```python
from build123d import *

# Parameters (mm, degrees)
BOSS_EXTRUDE1_DEPTH      = 3.175
BOSS_EXTRUDE1_DEPTH_BACK = 3.175
SKETCH1_R                = 4.178670833


with BuildPart() as part:
    # Sketch1 → Boss-Extrude1 (new, two sides: drawn at the far end of the back side and taken through both)
    with BuildSketch(Plane.XY.offset(-BOSS_EXTRUDE1_DEPTH_BACK)):
        with BuildLine():
            Line((596.301932932, 140.061825094), (593.775672351, 134.913286528))
            Line((593.775672351, 134.913286528), (596.301932932, 127.519508045))
            Line((596.301932932, 127.519508045), (596.301932932, 112.761180415))
            Line((596.301932932, 112.761180415), (620.507043959, 121.0314333))
            Line((620.507043959, 121.0314333), (621.935426787, 129.559046913))
            ThreePointArc((621.935426787, 129.559046913), (624.139317927, 134.860628873), (628.452705625, 138.649902417))
            ThreePointArc((628.452705625, 138.649902417), (629.422874429, 139.237084375), (630.327572389, 139.920847318))
            Line((630.327572389, 139.920847318), (641.475190915, 144.713939185))
            Line((641.475190915, 144.713939185), (645.828084101, 149.293372969))
            Line((645.828084101, 149.293372969), (645.073577651, 155.192660049))
            Line((645.073577651, 155.192660049), (642.120102738, 151.018989056))
            Line((642.120102738, 151.018989056), (637.784779863, 151.018989056))
            Line((637.784779863, 151.018989056), (631.886802035, 155.192660049))
            ThreePointArc((631.886802035, 155.192660049), (622.162679723, 159.329151932), (613.427511309, 153.382223935))
            ThreePointArc((613.427511309, 153.382223935), (611.595219928, 150.709853801), (609.146322902, 148.588119322))
            Line((609.146322902, 148.588119322), (596.301932932, 140.061825094))
        make_face()
        with Locations((623.238490422, 148.360136067)):
            Circle(SKETCH1_R, mode=Mode.SUBTRACT)
    extrude(amount=BOSS_EXTRUDE1_DEPTH + BOSS_EXTRUDE1_DEPTH_BACK)


solid = part.part
```
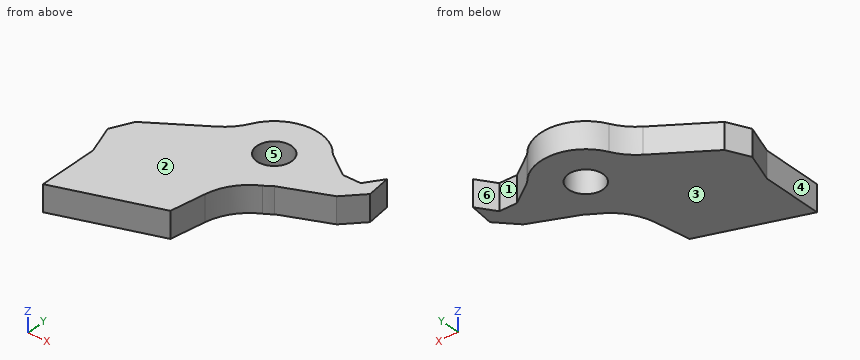
The model under review builds one solid part; all positions refer to its coordinate system, in mm. Face numbers are marked on the shaded views. A direction names the side the tool comes from. Round coordinates to 2 decimals unless told otherwise and drop trailing zeros. Order: outer loops, then holes, each group sorted by start corner. A loop starts at its lowest first (then second) coordinate and runs counter-clockwise, first axis right, second up. Notation, with made-up numbers: (-34, 76) - (22, 76) arc R27 cw to (22, 102) - close; hole circle Ø10 at (5, 15). An arc over 180 degrees is marked (long way). Answer in a Markdown table with one row per item.
(1) Mouldability with a two-part tool opening along X and no side actions: class the marked faces 3, 4, 5 and 6 as released by +X, released by -X, zero draft, split by the parting line, or undercut.
Result set:
| item | result |
|---|---|
| face 3 | zero draft |
| face 4 | released by -X |
| face 5 | undercut |
| face 6 | undercut |
(2) For line 1 (Y direction, x = 625, z = 0.25); line 2 (Y direction, x = 624.5, z = -0.25); line 3 (X direction, y = 147, z = -2.5), list the stretches that pass through material, from the lowest coordinate up. Write a range as from..to.
Result set:
| item | result |
|---|---|
| line 1 | y = 135.93..144.57, 152.15..159.24 |
| line 2 | y = 135.34..144.38, 152.34..159.31 |
| line 3 | x = 606.75..619.29, 627.19..643.65 |
(3) Take a section at A-A on x = 622.5. Write out the cut boundary in (y, z) (3 decimals), plus the area to 3 significant figures.
Result set:
| item | result |
|---|---|
| outline | (131.73, -3.175) - (144.247, -3.175) - (144.247, 3.175) - (131.73, 3.175) - close; (152.473, -3.175) - (159.357, -3.175) - (159.357, 3.175) - (152.473, 3.175) - close |
| area | 123 mm2 |
(4) Take a section at D-D on x = 610. Write out the cut boundary in (y, z) (3 decimals), plus the area to 3 significant figures.
Result set:
| item | result |
|---|---|
| outline | (117.441, -3.175) - (149.207, -3.175) - (149.207, 3.175) - (117.441, 3.175) - close |
| area | 202 mm2 |
(5) Machinability: for the marked faces 1 and 2, which of the approach directions +Z, -Z, +X, -X, +Y, -Y give a long, thin tool a straight path to every point of the face, cutting with its end or side? Answer none if there is none.
Result set:
| item | result |
|---|---|
| face 1 | +Z, -Z, +Y |
| face 2 | +Z, +X, -X, +Y, -Y |
(6) Clearance check with flat-ended pins moving along their axes: P1, Ø2, axis at y = 143, z = -2, coming from the -X side; P2, Ø2, axis at y = 130.5, z = -1.5, coming from the +X side; P3, Ø7.5, axis at x = 623.24, y = 148.36, coming from the -Z side; P4, Ø3, axis at y = 128, z = 2.5, coming from the -X side. State where each tip first meets the part, or that it passes through.
Result set:
| item | result |
|---|---|
| P1 | stops at x = 599.22 |
| P2 | stops at x = 622.42 |
| P3 | passes through |
| P4 | stops at x = 595.63 |
(7) Take a section at B-B on y = 145.5. Write out the cut boundary in (x, z) (3 decimals).
Result set:
| item | result |
|---|---|
| outline | (604.494, -3.175) - (620.192, -3.175) - (620.192, 3.175) - (604.494, 3.175) - close; (626.285, -3.175) - (642.222, -3.175) - (642.222, 3.175) - (626.285, 3.175) - close |
(8) Take a section at C-C on z = 1.75. Write out the cut boundary in (x, y).
Result set:
| item | result |
|---|---|
| outline | (593.78, 134.91) - (596.3, 127.52) - (596.3, 112.76) - (620.51, 121.03) - (621.94, 129.56) arc R12.7 cw to (628.45, 138.65) arc R11.02 ccw to (630.33, 139.92) - (641.48, 144.71) - (645.83, 149.29) - (645.07, 155.19) - (642.12, 151.02) - (637.78, 151.02) - (631.89, 155.19) arc R11.02 ccw to (613.43, 153.38) arc R12.7 cw to (609.15, 148.59) - (596.3, 140.06) - close; hole circle Ø8.36 at (623.24, 148.36) |
